```python
from build123d import *

# Parameters (mm, degrees)
SKETCH1_R           = 12.7
SKETCH1_R_2         = 4.445
BOSS_EXTRUDE2_DEPTH = 19.05


with BuildPart() as part:
    # Sketch1 → Boss-Extrude2 (new body)
    with BuildSketch(Plane(origin=(0, 0, 0), x_dir=(1, 0, 0), z_dir=(0, 1, 0))):
        with BuildLine():
            Line((6.178378378, -18.02027027), (57.15, -9.525))
            ThreePointArc((57.15, -9.525), (66.675, 0), (57.15, 9.525))
            Line((57.15, 9.525), (6.178378378, 18.02027027))
            ThreePointArc((6.178378378, 18.02027027), (-19.05, 0), (6.178378378, -18.02027027))
        make_face()
        with Locations(Location((0, 0, 0), (0, 0, 270))):
            Circle(SKETCH1_R, mode=Mode.SUBTRACT)
        with BuildLine():
            ThreePointArc((22.86, 5.054447816), (23.982759705, 7.477036261), (26.556966785, 8.186248525))
            Line((26.556966785, 8.186248525), (39.256966785, 6.069581858))
            ThreePointArc((39.256966785, 6.069581858), (41.157588444, 4.990021445), (41.91, 2.93778115))
            Line((41.91, 2.93778115), (41.91, -2.93778115))
            ThreePointArc((41.91, -2.93778115), (41.157588444, -4.990021445), (39.256966785, -6.069581858))
            Line((39.256966785, -6.069581858), (26.556966785, -8.186248525))
            ThreePointArc((26.556966785, -8.186248525), (23.982759705, -7.477036261), (22.86, -5.054447816))
            Line((22.86, -5.054447816), (22.86, 5.054447816))
        make_face(mode=Mode.SUBTRACT)
        with Locations(Location((57.15, 0, 0), (0, 0, 270))):
            Circle(SKETCH1_R_2, mode=Mode.SUBTRACT)
    extrude(amount=BOSS_EXTRUDE2_DEPTH)


solid = part.part
```
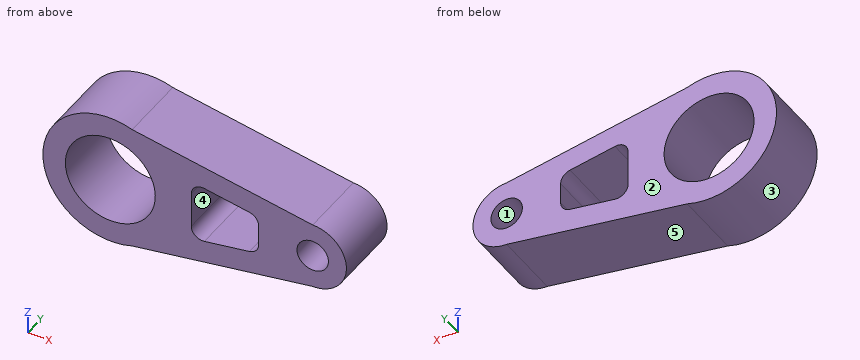
The model under review builds one solid part; all positions refer to its coordinate system, in mm. Face numbers are marked on the shaded views. A direction names the side the tool comes from. Round coordinates to 2 decimals unless told otherwise and drop trailing zeros. Loops run counter-clockwise (first coordinate to the right, second up) from the corner with the lowest first, then second, coordinate; pieces in that order, holes last.
Item 1: Take a section at C-C (z = -2). Write out the cut boundary in (x, y), then the cut area to 3 significant figures.
Determined:
outline: (-18.94, 0) - (-12.54, 0) - (-12.54, 19.05) - (-18.94, 19.05) - close; (12.54, 0) - (22.86, 0) - (22.86, 19.05) - (12.54, 19.05) - close; (41.91, 0) - (53.18, 0) - (53.18, 19.05) - (41.91, 19.05) - close; (61.12, 0) - (66.46, 0) - (66.46, 19.05) - (61.12, 19.05) - close
area: 635 mm2
Item 2: For the marked faces 4 and 5, list the 3-axis set-ups (+Z, -Z, +X, -X, +Y, -Y) from which the entire face can be reached by the end or side of a thin tool; tool diameter is ignored.
Determined:
face 4: +Y, -Y
face 5: -Z, +X, +Y, -Y
Item 3: Mouldability with a two-part tool opening along X and no side actions: class the marked faces 1, 2 and 3 as released by +X, released by -X, zero draft, split by the parting line, or undercut.
Determined:
face 1: undercut
face 2: zero draft
face 3: split by the parting line
Item 4: Take a section at B-B (y = 13). Write out the cut boundary in (x, z) (3 decimals), then the cut area to 3 significant figures.
Determined:
outline: (6.178, -18.02) - (57.15, -9.525) arc R9.525 ccw to (57.15, 9.525) - (6.178, 18.02) arc R19.05 ccw (long way) to start; hole circle Ø25.4 at (0, 0); hole (22.86, -5.054) arc R3.175 ccw to (26.557, -8.186) - (39.257, -6.07) arc R3.175 ccw to (41.91, -2.938) - (41.91, 2.938) arc R3.175 ccw to (39.257, 6.07) - (26.557, 8.186) arc R3.175 ccw to (22.86, 5.054) - close; hole circle Ø8.89 at (57.15, 0)
area: 1,510 mm2
Item 5: For line 1 (X direction, y = 4, z = 0) (3 decimals); line 2 (X direction, y = 8.5, z = 4); line 3 (X direction, y = 11.25, z = -5), list the stretches that pass through material, from the lowest coordinate up.
Determined:
line 1: x = -19.05 to -12.7, 12.7 to 22.86, 41.91 to 52.705, 61.595 to 66.675
line 2: x = -18.63 to -12.05, 12.05 to 22.86, 41.73 to 55.21, 59.09 to 65.79
line 3: x = -18.38 to -11.67, 11.67 to 22.86, 41.15 to 65.26
Item 6: Take a section at D-D (x = 41). Write out the cut boundary in (y, z).
Determined:
outline: (0, -12.22) - (19.05, -12.22) - (19.05, -5.16) - (0, -5.16) - close; (0, 5.16) - (19.05, 5.16) - (19.05, 12.22) - (0, 12.22) - close
Item 7: Take a section at A-A (x = 0). Write out the cut boundary in (y, z).
Determined:
outline: (0, -19.05) - (19.05, -19.05) - (19.05, -12.7) - (0, -12.7) - close; (0, 12.7) - (19.05, 12.7) - (19.05, 19.05) - (0, 19.05) - close
Item 8: Clearance check with flat-ended pins moving along their axes: pin 1 Ø4 at (y, z) = (16, 11.5) entering from -X; pin 2 Ø3 at (x, y) = (32.5, 15.5) entering from -Z; pin 3 Ø1.5 at (y, z) = (14, -3.5) entering from +X. State where each tip first meets the part, or that it passes through.
Determined:
pin 1: stops at x = -16.51
pin 2: stops at z = -13.88
pin 3: stops at x = 66.27
